Autodesk Inventor part; units mm, degrees
ref_plane "YZ Plane" through (0, 0, 0) normal (1, 0, 0) x (0, 1, 0)
ref_plane "XZ Plane" through (0, 0, 0) normal (0, 1, 0) x (-1, 0, 0)
ref_plane "XY Plane" through (0, 0, 0) normal (0, 0, 1) x (1, 0, 0)
sketch "Sketch2" plane through (0, 0, 0) normal (0, 1, 0) x (-1, 0, 0)
  line L0 (-50, -100) -> (50, -100)
  line L1 (50, -100) -> (50, 100)
  line L2 (50, 100) -> (-50, 100)
  line L3 (-50, 100) -> (-50, -100)
  line L4 (-50, -100) -> (50, 100) construction
  line L5 (50, -100) -> (-50, 100) construction
  point P0 (0, 0)
  dimension "d0" = 200
  dimension "d1" = 100
extrude "Extrusion1" add sketch "Sketch2" along normal blind 2
sketch "Sketch3" plane through (0, 2, 0) normal (0, 1, 0) x (1, 0, 0)
  circle A0 centre (33.1152, 84.1449) radius 10
  circle A1 centre (33.1152, 59.7195) radius 10
  circle A2 centre (33.1152, 33.634) radius 10
  point P0 (0, 0)
  dimension "d4" = 20
  dimension "d5" = 20
  dimension "d6" = 20
extrude "Extrusion2" add sketch "Sketch3" along normal blind 45
sketch "Sketch4" plane through (0, 2, 0) normal (0, 1, 0) x (1, 0, 0)
  line L0 (-25, -99) -> (-5, -99)
  line L1 (-5, -99) -> (-5, -69)
  line L2 (-5, -69) -> (-25, -69)
  line L3 (-25, -69) -> (-25, -99)
  line L4 (-25, -99) -> (-5, -69) construction
  line L5 (-5, -99) -> (-25, -69) construction
  line L6 (-50, 100) -> (-50, -100)
  line L7 (-50, -100) -> (50, -100)
  point P0 (0, 0)
  point P1 (-15, -84)
  dimension "d9" = 25
  dimension "d10" = 45
  dimension "d11" = 30
  dimension "d12" = 1
extrude "Extrusion3" add sketch "Sketch4" along normal blind 2
equation "\"BendRadius\" = Thickness"
equation "\"BendReliefWidth\" = Thickness"
equation "\"BendReliefDepth\" = 0.5 * Thickness"
equation "\"CornerReliefSize\" = 4 * Thickness"
equation "\"MinimumRemnant\" = 2 * Thickness"
equation "\"TransitionRadius\" = BendRadius"
equation "\"JacobiRadiusSize\" = BendRadius"
equation "\"GapSize\" = Thickness"
properties part number "modelo placa"
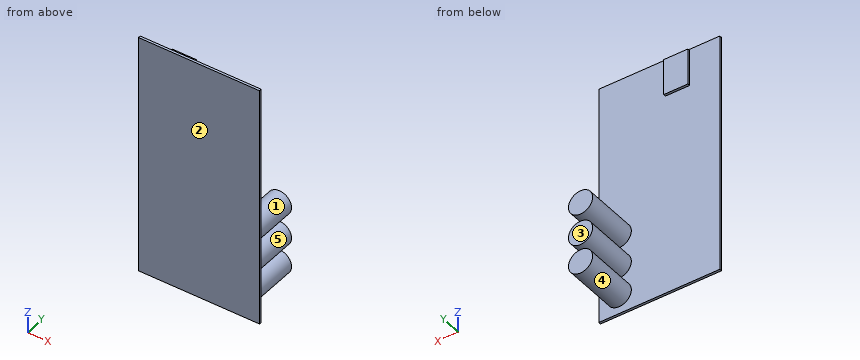
The model under review builds one solid part; all positions refer to its coordinate system, in mm. Face numbers are marked on the shaded views. A direction names the side the tool comes from. Coordinates: 2 decimals unless noted, no trailing zeros. Order: outer loops, then holes, each group sorted by start corner. A loop starts at its lowest first (then second) coordinate and runs counter-clockwise, first axis right, second up. Notation, with made-up numbers: (-10, -8.5) -> (15, -8.5) arc R8 ccw to (15, -2.5) -> close; hole circle Ø5 at (79.25, 70.5). An arc over 180 degrees is marked (long way). Answer in a Markdown table with one row per item. Add a question column.
Item 1: Machinability: for the marked faces 1 and 2, which of the approach directions +Z, -Z, +X, -X, +Y, -Y give a long, thin tool a straight path to every point of the face, cutting with its end or side? Answer none if there is none.
Item 2: We need section D-D on x = 28. Write out the cut boundary in (y, z), plus the area to 3 significant figures.
Item 3: We need section A-A on x = -13. Write out the cut boundary in (y, z).
Item 4: To check wall thickness, follow probe 1 along Y at (x, z) = (-14, 4); probe 2 along Z at (x, y) = (-22.5, 3); probe 3 along X at (y, z) = (10, -84.5). State the ranges of each line that lie inside material, in increasing order.
Item 5: We need section B-B on z = 71.5. Write out the cut boundary in (x, y).
Item 6: Clearance check with flat-ended pins moving along their axes: pin 1 (0.6 mm diameter, centred on y = 3, z = 82, fed in from -X); pin 2 (2 mm diameter, centred on x = 3, z = -30, fed in from +Y); pin 3 (16 mm diameter, centred on x = -10.5, z = 91.5, fed in from +Y). State where each tip first meets the part, or that it passes through.
Item 7: Mouldability with a two-part tool opening along Z and no side actions: class the marked faces 3, 4 and 5 as +Z half, -Z half, draft (parallel to the pull), parting line (faces both ways), or undercut.
Item 8: We need section C-C on y = 22. Write out the cut boundary in (x, z), plus the area to 3 significant figures.
Final values:
| question | item | result |
|---|---|---|
| 1 | face 1 | +Y |
| 1 | face 2 | +Z, -Z, +X, -X, -Y |
| 2 | outline | (0, -100) -> (2, -100) -> (2, -92.74) -> (47, -92.74) -> (47, -75.55) -> (2, -75.55) -> (2, -68.31) -> (47, -68.31) -> (47, -51.13) -> (2, -51.13) -> (2, -42.23) -> (47, -42.23) -> (47, -25.04) -> (2, -25.04) -> (2, 100) -> (0, 100) -> close |
| 2 | area | 2,720 mm2 |
| 3 | outline | (0, -100) -> (2, -100) -> (2, 69) -> (4, 69) -> (4, 99) -> (2, 99) -> (2, 100) -> (0, 100) -> close |
| 4 | probe 1 | y = 0 to 2 |
| 4 | probe 2 | z = 69 to 99 |
| 4 | probe 3 | x = 23.12 to 43.11 |
| 5 | outline | (-50, 0) -> (50, 0) -> (50, 2) -> (-5, 2) -> (-5, 4) -> (-25, 4) -> (-25, 2) -> (-50, 2) -> close |
| 6 | pin 1 | stops at x = -25 |
| 6 | pin 2 | stops at y = 2 |
| 6 | pin 3 | stops at y = 4 |
| 7 | face 3 | draft |
| 7 | face 4 | undercut |
| 7 | face 5 | undercut |
| 8 | outline | circle Ø20 at (33.12, -84.14); circle Ø20 at (33.12, -59.72); circle Ø20 at (33.12, -33.63) |
| 8 | area | 942 mm2 |
